The listing builds one solid part. Answer for the finished solid, in the listing's coordinates (mm). A direction names the side the tool comes from. Round coordinates to 2 decimals unless told otherwise and drop trailing zeros. Write each question's results on one line, items separated by ' | '. Start each with the question number.
(1) Determine the mould class of faces 3 (the face through (15, 0, 15)), 4 (the face through (29.414, -1.521, 0.481)), 5 (the face through (-10.21, -1.48, -32.43)) for opening direction Z: released by +Z, released by -Z, zero draft, split by the parting line, or undercut.
(2) The part is cut by section A-A (z = 0). Count the separate pieces of the cut face and the enclosed holes in it, plus the area to 3 significant figures.
(3) Flat-ended cylindrical pins translate along their axes: pin 1 (6 mm diameter, centred on y = -5, z = 21, fed in from +X); pin 2 (10 mm diameter, centred on x = -10.5, z = 17.5, fed in from -Y); pin 3 (1 mm diameter, centred on y = -4, z = 8, fed in from -X); pin 4 (3 mm diameter, centred on x = -27.89, z = 0, fed in from +Y). Find the tip coordinate at first contact, or state that the pin passes through.
(4) For faces 1 (the face through (0.481, -1.521, -29.414)), 2 (the face through (22, -3, 0)), determine the directions among +Z, -Z, +X, -X, +Y, -Y from which every point of the face is accessible in a straight line to the end or side of a thin tool.
(5) Straight lines are drawn through the part: probe 1 along Y at (x, z) = (-21.5, 9); probe 2 along X at (y, z) = (-1.5, 1); probe 3 along X at (y, z) = (-1, -27.5). For each, find the intervals that lie inside material, in ascending order.
```python
from build123d import *

# Parameters (mm, degrees)
SKETCH3_W          = 13.453428953
SKETCH3_H          = 3
FILLET1_R          = 1.5
SKETCH4_R          = 1.6
CUT_EXTRUDE1_DEPTH = 51.079936266
CIRPATTERN1_COUNT  = 4


with BuildPart() as part:
    # Sketch1 → Revolve1 (revolve)
    with BuildSketch(Plane.XY, mode=Mode.PRIVATE) as revolve1_sk:
        with BuildLine():
            Line((0, -17), (0, -14))
            add(Edge.make_bspline(
                [(0, -14), (16.389539142, -14), (17.019517421, -6.054809845), (18, 0)],
                knots=[0, 0, 0, 0, 1, 1, 1, 1], degree=3))
            Line((18, 0), (20.961422891, 0))
            Line((20.961422891, 0), (20.961422891, -0.479556523))
            add(Edge.make_bspline(
                [(0, -17), (0.528573753, -17), (1.605388754, -16.983569549), (3.600168077, -16.886379692), (5.915984959, -16.646675198), (8.402442715, -16.175166648), (11.369715767, -15.30568509), (14.467863823, -13.768247798), (17.226954494, -11.272431323), (19.016831185, -8.41451175), (20.041971454, -5.53113124), (20.509739393, -3.277227242), (20.784228644, -1.605380322), (20.899427173, -0.862400942), (20.961422891, -0.479556523)],
                knots=[0, 0, 0, 0, 0.03125, 0.0625, 0.125, 0.1875, 0.25, 0.375, 0.5, 0.625, 0.75, 0.875, 0.9375, 1, 1, 1, 1], degree=3))
        make_face()
    revolve(revolve1_sk.sketch.rotate(Axis((0, -17, 0), (0, 1, 0)), 90), axis=Axis((0, -17, 0), (0, 1, 0)))

    # Sketch3 → Revolve2 (revolve)
    with BuildSketch(Plane.XY, mode=Mode.PRIVATE) as revolve2_sk:
        with Locations((27.273285524, -1.5)):
            Rectangle(SKETCH3_W, SKETCH3_H)
    revolve(revolve2_sk.sketch.rotate(Axis((0, 0, 0), (0, 1, 0)), 90), axis=Axis((0, 0, 0), (0, 1, 0)))

    # Fillet1
    fillet1_edges = [part.edges().sort_by_distance(p)[0] for p in [
        (0, -3, 20.546571047),
    ]]
    fillet(fillet1_edges, radius=FILLET1_R)

    # Sketch4 → Cut-Extrude1 (cut, through all)
    with BuildSketch(Plane.XZ.offset(3)):
        with Locations(Location((0, -27.888022688, 0), (0, 0, 270))):
            Circle(SKETCH4_R)
    cut_extrude1 = extrude(amount=-CUT_EXTRUDE1_DEPTH, mode=Mode.SUBTRACT)

    # CirPattern1: Cut-Extrude1 ×4 about axis
    cirpattern1_axis = Axis((0, 0, 0), (0, 1, 0))
    for i in range(1, CIRPATTERN1_COUNT):
        add(cut_extrude1.rotate(cirpattern1_axis, i * 360 / CIRPATTERN1_COUNT), mode=Mode.SUBTRACT)


solid = part.part
```
Checked values:
1) face 3: zero draft | face 4: undercut | face 5: split by the parting line
2) separate pieces: 3 | enclosed holes: 0 | area: 230 mm2
3) pin 1: stops at x = 28.35 | pin 2: stops at y = -12.84 | pin 3: stops at x = -19.09 | pin 4: passes through
4) face 1: +Y, -Y | face 2: -Y
5) probe 1: y = -3 to 0 | probe 2: x = -33.99 to -29.14, -26.64 to -17.73, 17.73 to 26.64, 29.14 to 33.99 | probe 3: x = -19.99 to -1.55, 1.55 to 19.99
